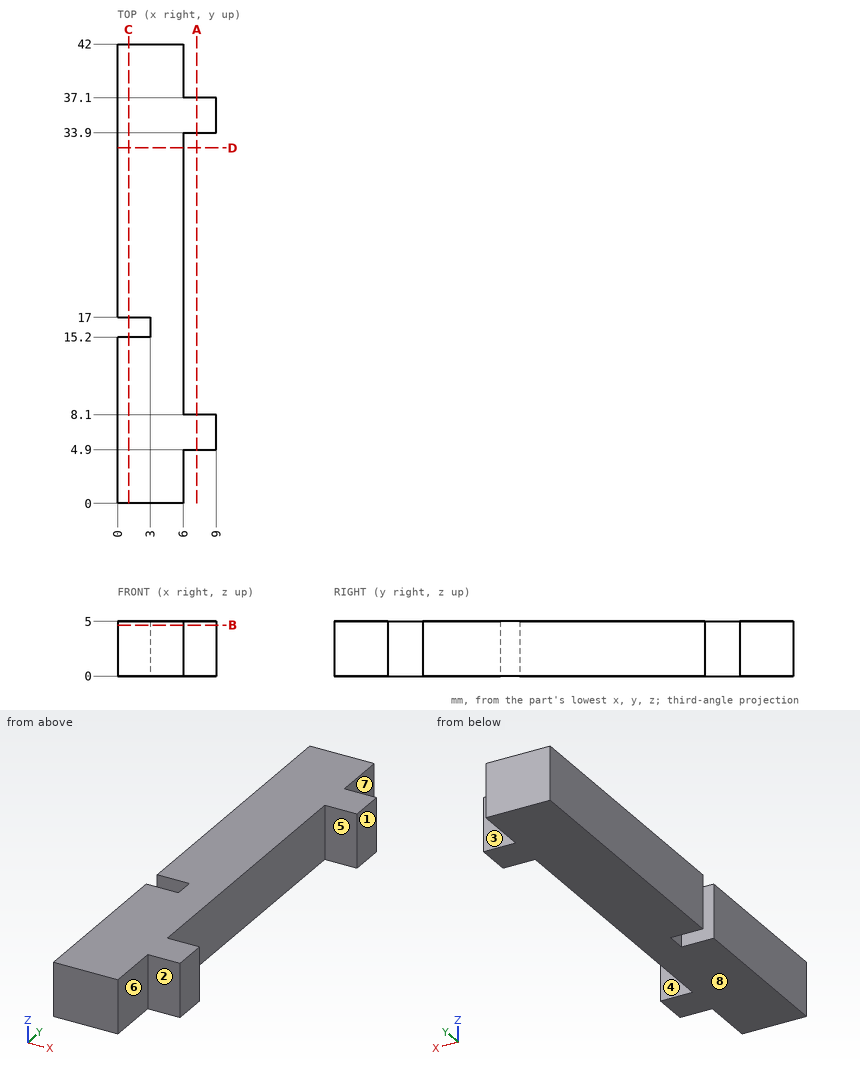
Drawing for the job (mm, zero at the part's lowest x, y, z). A direction names the side the tool comes from. Coordinates: 2 decimals unless noted, no trailing zeros. Write each loop counter-clockwise with the first axis right and the second up, starting at its lowest first coordinate (ties: lowest second). Pieces come first, ordered by that corner, then holes. Notation, with made-up numbers: (33, 48) -> (77, 48) arc R17 cw to (77, 64) -> close; hole circle Ø7 at (75.5, -35.75). An arc over 180 degrees is marked (long way). One line per item, written item: value. Start each with the question number.
1) Slice it at A-A on x = 7.25. Write the cut outline in (y, z).
2) Probe probe 1 along Y at (x, z) = (7, 3.1); probe 2 along Y at (x, z) = (2.25, 4.5); probe 3 along X at (y, z) = (28, 0.6). List the from-to ranges inside material, lowest first.
3) Flat gauge pins, fed straight in: pin 1 Ø2.5 at (x, z) = (1, 2.5) entering from -Y; pin 2 Ø1.5 at (y, z) = (3, 2.5) entering from +X. Where does each tip first touch, or does it go through?
4) Pull direction Y, two halves, no side cores. Call the marked faces 1, 2, 3 and 4: +Y half, -Y half, draft (parallel to the pull), parting line (faces both ways), or undercut.
5) Slice it at B-B on z = 4.65. Write the cut outline in (x, y), then the cut area to 3 significant figures.
6) Slice it at D-D on y = 32.5. Write the cut outline in (x, z).
7) Which spindle directions (+Z, -Z, +X, -X, +Y, -Y) get a long thin tool onto all of the face, cutting with end or side? Do the marked faces 5, 6, 7 and 8. Say none if no direction does.
8) Slice it at C-C on x = 1. Write the cut outline in (y, z), then the cut area to 3 significant figures.
Answers follow:
1. outline: (4.9, 0) -> (8.1, 0) -> (8.1, 5) -> (4.9, 5) -> close; (33.9, 0) -> (37.1, 0) -> (37.1, 5) -> (33.9, 5) -> close
2. probe 1: 4.9 to 8.1, 33.9 to 37.1
2. probe 2: 0 to 15.2, 17 to 42
2. probe 3: 0 to 6
3. pin 1: y = 0
3. pin 2: x = 6
4. face 1: draft
4. face 2: -Y half
4. face 3: +Y half
4. face 4: undercut
5. outline: (0, 0) -> (6, 0) -> (6, 4.9) -> (9, 4.9) -> (9, 8.1) -> (6, 8.1) -> (6, 33.9) -> (9, 33.9) -> (9, 37.1) -> (6, 37.1) -> (6, 42) -> (0, 42) -> (0, 17) -> (3, 17) -> (3, 15.2) -> (0, 15.2) -> close
5. area: 266 mm2
6. outline: (0, 0) -> (6, 0) -> (6, 5) -> (0, 5) -> close
7. face 5: +Z, -Z, +X
7. face 6: +Z, -Z, +X, -Y
7. face 7: +Z, -Z, +X, +Y
7. face 8: -Z, +X, -X, +Y, -Y
8. outline: (0, 0) -> (15.2, 0) -> (15.2, 5) -> (0, 5) -> close; (17, 0) -> (42, 0) -> (42, 5) -> (17, 5) -> close
8. area: 201 mm2
